```python
from build123d import *

# Parameters (mm, degrees)
F0_W      = 57.15
F0_H      = 88.9
F1_DEPTH  = 3.175
F2_W      = 3.175
F2_H      = 88.9
F3_DEPTH  = 50.8
F4_W      = 3.175
F4_H      = 88.9
F5_DEPTH  = 50.8
F6_W      = 3.175
F6_H      = 88.9
F7_DEPTH  = 50.8
F7_FACE_W = 3.175
F7_FACE_H = 88.9
F8_DEPTH  = 50.8
F9_W      = 3.175
F9_H      = 88.9
F10_DEPTH = 23.8125
F11_W     = 50.8
F11_H     = 88.9
F12_DEPTH = 3.175
F13_W     = 3.175
F13_H     = 88.9
F14_DEPTH = 23.8125
F15_W     = 57.15
F15_H     = 88.9
F16_DEPTH = 3.175
F17_W     = 56.964433
F17_H     = 57.15
F18_DEPTH = 3.175


with BuildPart() as f1:
    # F0 (on Front) → F1 (new body)
    with BuildSketch(Plane.XZ):
        Rectangle(F0_W, F0_H)
    extrude(amount=F1_DEPTH)

    # F2 (on face) → F3 (join)
    with BuildSketch(Plane(origin=(0, 0, 0), x_dir=(-1, 0, 0), z_dir=(0, 1, 0))):
        with Locations((-26.9875, 0)):
            Rectangle(F2_W, F2_H)
    extrude(amount=F3_DEPTH)

    # F4 (on face) → F5 (join)
    with BuildSketch(Plane(origin=(0, 0, 0), x_dir=(-1, 0, 0), z_dir=(0, 1, 0))):
        with Locations((26.9875, 0)):
            Rectangle(F4_W, F4_H)
    extrude(amount=F5_DEPTH)

    # F6 (on face) → F7 (join)
    with BuildSketch(Plane(origin=(0, 0, 0), x_dir=(-1, 0, 0), z_dir=(0, 1, 0))):
        Rectangle(F6_W, F6_H)
    extrude(amount=F7_DEPTH)

    # F7_face (on face) → F8 (cut)
    with BuildSketch(Plane(origin=(0, 50.8, 0), x_dir=(-1, 0, 0), z_dir=(0, 1, 0))):
        Rectangle(F7_FACE_W, F7_FACE_H)
    extrude(amount=-F8_DEPTH, mode=Mode.SUBTRACT)



with BuildPart() as f10:
    # F9 (on face) → F10 (new body)
    with BuildSketch(Plane(origin=(0, 26.9875, 0), x_dir=(-1, 0, 0), z_dir=(0, 1, 0))):
        Rectangle(F9_W, F9_H)
    extrude(amount=F10_DEPTH)


with BuildPart() as f1_1:
    add(f1.part)

    add(f10.part)  # F12 merges F10
    # F11 (on face) → F12 (join)
    with BuildSketch(Plane(origin=(0, 23.8125, 0), x_dir=(-1, 0, 0), z_dir=(0, 1, 0))):
        Rectangle(F11_W, F11_H)
    extrude(amount=F12_DEPTH)

    # F13 (on face) → F14 (join)
    with BuildSketch(Plane(origin=(0, 0, 0), x_dir=(-1, 0, 0), z_dir=(0, 1, 0))):
        Rectangle(F13_W, F13_H)
    extrude(amount=F14_DEPTH)

    # F15 (on face) → F16 (join)
    with BuildSketch(Plane(origin=(0, 50.8, 0), x_dir=(-1, 0, 0), z_dir=(0, 1, 0))):
        Rectangle(F15_W, F15_H)
    extrude(amount=F16_DEPTH)

    # F17 (on face) → F18 (join)
    with BuildSketch(Plane(origin=(0, 0, -44.45), x_dir=(1, 0, 0), z_dir=(0, 0, -1))):
        with Locations((-0.092783, -25.4)):
            Rectangle(F17_W, F17_H)
    extrude(amount=F18_DEPTH)


solid = f1_1.part
```
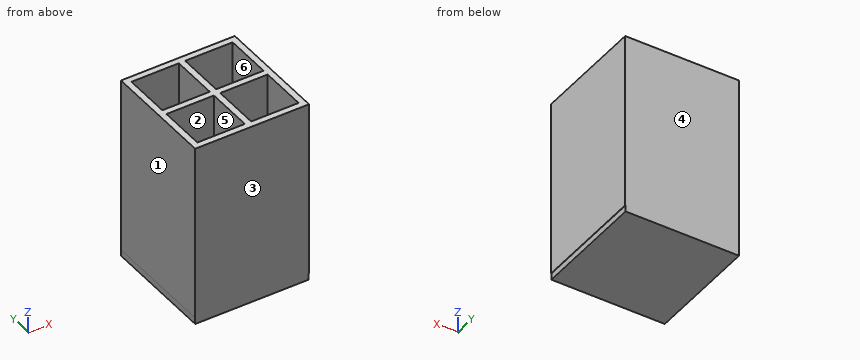
Input: part model. Units: mm. Frame: model coordinates. Face numbers are marked on the shaded views. A direction names the side the tool comes from. Coordinates: 2 decimals unless noted, no trailing zeros. Loops run counter-clockwise (first coordinate to the right, second up) from the corner with the lowest first, then second, coordinate; pieces in that order, holes last. Notation, with made-up numbers: M 67.25,15 L 124.25,15 A34 cw 124.25,46 Z; hole C 10.25,-5 d5. An arc over 180 degrees is marked long. One line per item, written item: value.
(1) Pin query (flat end, axial travel): pin 1 (12 mm diameter, centred on x = -10.5, y = 39, fed in from +Z); pin 2 (1.6 mm diameter, centred on y = 26.5, z = -45.5, fed in from +X). Return the tip coordinate at first contact, or that it passes through.
Filled in:
pin 1: z = -44.45
pin 2: x = 28.39
(2) Line query: line 1 along Y through (x, z) = (-10, -15.5) (1 decimal); line 2 along X through (y, z) = (40.5, -17.5) (1 decimal); line 3 along Z through (x, y) = (11.5, 14.5) (3 decimals). Output: solid intervals per line, ascending. Write a range as from..to.
Filled in:
line 1: -3.2..0, 23.8..27, 50.8..54
line 2: -28.6..-25.4, -1.6..1.6, 25.4..28.6
line 3: -47.625..-44.45
(3) Section A-A (z = -2). Output: boundary loops of the cut face in (x, y) (1 decimal), and give its area (3 significant figures).
Filled in:
outline: M -28.6,-3.2 L 28.6,-3.2 L 28.6,54 L -28.6,54 Z; hole M -25.4,0 L -1.6,0 L -1.6,23.8 L -25.4,23.8 Z; hole M -25.4,27 L -1.6,27 L -1.6,50.8 L -25.4,50.8 Z; hole M 1.6,0 L 25.4,0 L 25.4,23.8 L 1.6,23.8 Z; hole M 1.6,27 L 25.4,27 L 25.4,50.8 L 1.6,50.8 Z
area: 998 mm^2
(4) Pull-direction query (Y, two-part tool) for the marked faces 3, 4, 5 and 6; classes: +Y half, -Y half, draft (parallel to the pull), parting line (faces both ways), or undercut.
Filled in:
face 3: -Y half
face 4: +Y half
face 5: undercut
face 6: undercut
(5) Reachability of the marked faces 1 and 2 from +Z, -Z, +X, -X, +Y, -Y: full face, straight path, thin tool, end or side. Return the list, or none.
Filled in:
face 1: +Z, -Z, -X, +Y, -Y
face 2: +Z
